from build123d import *

# Parameters (mm, degrees)
F0_W         = 31
F0_H         = 21
F1_DEPTH     = 3
F2_W         = 31
F2_H         = 14
F3_DEPTH     = 3
F4_W         = 25.4
F4_H         = 1.2
F5_DEPTH     = 25
F6_W         = 25.4
F6_H         = 19.5
F7_DEPTH     = 1
F8_R         = 0.59999
F9_R         = 2.6
F10_W        = 25.4
F10_H        = 0.75
F11_DEPTH    = 0.5
F12_T4_DEPTH = 25.4
F12_T9_DEPTH = 25.4
F13_R        = 2
F14_SIZE     = 0.99999
F15_R        = 2


# Not quite as in the source:
# - a fillet or chamfer that OpenCascade refuses, or shapes differently, is made with other operations: its cross-section is extruded or revolved along the edge and cut away or added
# - a fillet or chamfer is up to 0.001 mm smaller than in the source, because OpenCascade refuses the exact size


with BuildPart() as f1:
    # F0 (on Top) → F1 (new body)
    with BuildSketch(Plane.XY):
        Rectangle(F0_W, F0_H)
    extrude(amount=F1_DEPTH)

    # F2 (on face) → F3 (join)
    with BuildSketch(Plane.XY.offset(3)):
        with Locations((0, 3.5)):
            Rectangle(F2_W, F2_H)
    extrude(amount=F3_DEPTH)

    # F4 (on face) → F5 (cut)
    with BuildSketch(Plane.XZ.offset(3.5)):
        with Locations((0, 3.6)):
            Rectangle(F4_W, F4_H)
    extrude(amount=-F5_DEPTH, mode=Mode.SUBTRACT)

    # F6 (on face) → F7 (cut)
    with BuildSketch(Plane(origin=(0, 0, 0), x_dir=(1, 0, 0), z_dir=(0, 0, -1))):
        with Locations((0, -0.75)):
            Rectangle(F6_W, F6_H)
    extrude(amount=-F7_DEPTH, mode=Mode.SUBTRACT)

    # F8 (radius 0.6 in the source; OpenCascade refuses exactly that, so slightly less here)
    f8_edges = [f1.edges().sort_by_distance(p)[0] for p in [
        (12.7, 3.5, 4.2),
        (12.7, 3.5, 3),
        (-12.7, 3.5, 3),
        (-12.7, 3.5, 4.2),
    ]]
    fillet(f8_edges, radius=F8_R)

    # F9
    f9_edges = [f1.edges().sort_by_distance(p)[0] for p in [
        (-15.5, 3.5, 6),
        (15.5, 3.5, 6),
    ]]
    fillet(f9_edges, radius=F9_R)

    # F10 (on face) → F11 (join)
    with BuildSketch(Plane(origin=(0, 0, 1), x_dir=(1, 0, 0), z_dir=(0, 0, -1))):
        with Locations((0, -0.375)):
            Rectangle(F10_W, F10_H)
    extrude(amount=F11_DEPTH)

    # F12: chamfer of 0.5 on 2 edges, made by hand


with BuildPart() as f12_tool2:
    # F12_s3 → F12_t4 (new body)
    with BuildSketch(Plane.YZ.offset(12.7)):
        Polygon((0.5, 0.5), (0, 1), (0, 0.5), align=None)
    extrude(amount=-F12_T4_DEPTH)

    split(bisect_by=Plane.XY.offset(1), keep=Keep.BOTTOM)


with BuildPart() as f1_1:
    add(f1.part)

    # F12_t1: cut F12_tool2
    add(f12_tool2.part, mode=Mode.SUBTRACT)


with BuildPart() as f12_tool7:
    # F12_s8 → F12_t9 (new body)
    with BuildSketch(Plane.YZ.offset(-12.7)):
        Polygon((0.75, 1), (0.25, 0.5), (0.75, 0.5), align=None)
    extrude(amount=F12_T9_DEPTH)

    split(bisect_by=Plane.XY.offset(1), keep=Keep.BOTTOM)


with BuildPart() as f1_2:
    add(f1_1.part)

    # F12_t6: cut F12_tool7
    add(f12_tool7.part, mode=Mode.SUBTRACT)

    # F13
    f13_edges = [f1_2.edges().sort_by_distance(p)[0] for p in [
        (15.5, -10.5, 1.5),
        (-15.5, -10.5, 1.5),
    ]]
    fillet(f13_edges, radius=F13_R)

    # F14 (size 1 in the source; OpenCascade refuses exactly that, so slightly less here)
    f14_edges = [f1_2.edges().sort_by_distance(p)[0] for p in [
        (0, -9, 1),
    ]]
    chamfer(f14_edges, length=F14_SIZE)

    # F15
    f15_edges = [f1_2.edges().sort_by_distance(p)[0] for p in [
        (0, -10.5, 3),
    ]]
    fillet(f15_edges, radius=F15_R)


solid = f1_2.part
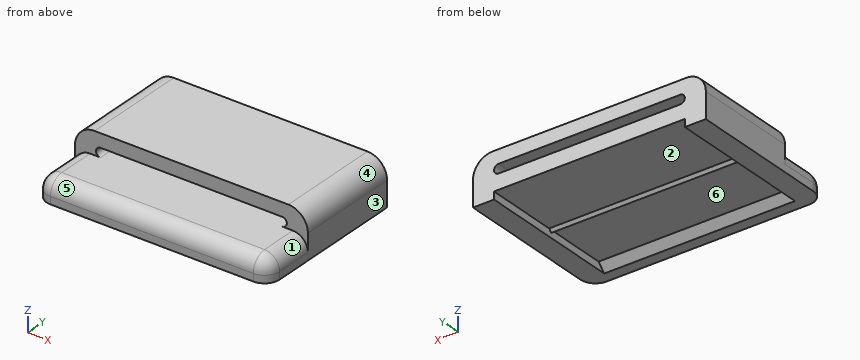
Input: part model. Units: mm. Frame: model coordinates. Face numbers are marked on the shaded views. A direction names the side the tool comes from. Round coordinates to 2 decimals unless told otherwise and drop trailing zeros. Loops run counter-clockwise (first coordinate to the right, second up) from the corner with the lowest first, then second, coordinate; pieces in that order, holes last. Notation, with made-up numbers: (30.5, 87.25) -> (86.5, 87.25) arc R22 ccw to (86.5, 106.25) -> close; hole circle Ø10 at (-39, 48.25). An arc over 180 degrees is marked (long way). Answer as a JSON object with one key per item and string values. Group by question number.
1) Ray query, L1, parallel to Z at x = -0.5, y = -3; L2, parallel to X at y = 1, z = 0.5; L3, parallel to Z at x = -13, y = -5.25. Return the intervals inside material, ascending.
2) Reachability of the marked faces 1, 2 and 3 from +Z, -Z, +X, -X, +Y, -Y: full face, straight path, thin tool, end or side. Return the list, or none.
3) Section query D-D on y = -6. Output: boundary loops of the cut face in (x, z).
4) Draft query along Y for the marked faces 4, 5 and 6. Return one class per face: +Y half, -Y half, draft (parallel to the pull), parting line (faces both ways), or undercut.
5) Section query C-C on z = 2.4. Output: boundary loops of the cut face in (x, y).
6) Pin query (flat end, axial travel): pin 1 (3 mm diameter, centred on x = 8.5, y = -4, fed in from -Z); pin 2 (1.5 mm diameter, centred on x = -4, z = 4, fed in from -Y). Return the tip coordinate at first contact, or that it passes through.
Reply:
{
 "1": {"L1": "z = 1 to 3, 4.2 to 6", "L2": "x = -15.5 to -12.7, 12.7 to 15.5", "L3": "z = 0 to 3"},
 "2": {"face 1": "+Z, +X, -Y", "face 2": "-Z, +Y", "face 3": "+Z, -Z, +X, +Y, -Y"},
 "3": {"outline": "(-15.5, 0) -> (-12.7, 0) -> (-12.7, 1) -> (12.7, 1) -> (12.7, 0) -> (15.5, 0) -> (15.5, 1) arc R2 ccw to (13.5, 3) -> (-13.5, 3) arc R2 ccw to (-15.5, 1) -> close"},
 "4": {"face 4": "draft", "face 5": "-Y half", "face 6": "undercut"},
 "5": {"outline": "(-15.5, -3.5) -> (-14.93, -3.5) -> (-14.93, -8.5) arc R1.43 ccw to (-13.5, -9.93) -> (13.5, -9.93) arc R1.43 ccw to (14.93, -8.5) -> (14.93, -3.5) -> (15.5, -3.5) -> (15.5, 10.5) -> (-15.5, 10.5) -> close"},
 "6": {"pin 1": "stops at z = 1", "pin 2": "stops at y = -3.5"}
}
